Verification items for this drawing (mm, ordinates from the low corner). A direction names the side the tool comes from. Give positions to 0.01 mm unless a question says otherwise; leave off trailing zeros. Write each loop counter-clockwise with the first axis right and the second up, starting at its lowest first coordinate (ties: lowest second). Pieces come first, ordered by that corner, then holes. Notation, with made-up numbers: (5, 59) -> (59, 59) arc R22 ccw to (59, 93) -> close; hole circle Ø4 at (68, 61). An arc over 180 degrees is marked (long way). Write item = value, one per line.
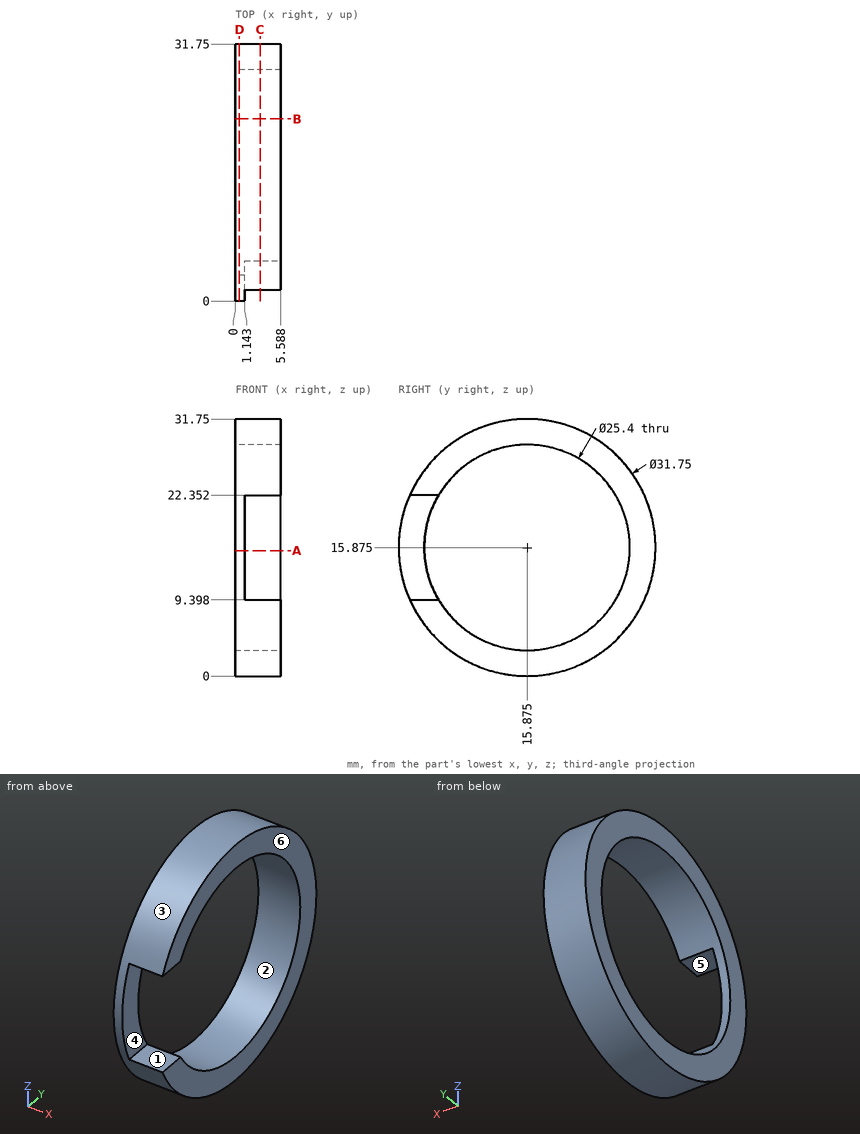
Item 1: Sectioned sample at B-B on y = 22.5. Record the cut outline in (x, z), then the cut area to 3 significant figures.
Response values:
outline = (0, 1.45) -> (5.59, 1.45) -> (5.59, 5.04) -> (0, 5.04) -> close; (0, 26.71) -> (5.59, 26.71) -> (5.59, 30.3) -> (0, 30.3) -> close
area = 40.1 mm^2
Item 2: Sectioned sample at C-C on x = 3.05. Record the cut outline in (y, z) (3 decimals), then the cut area to 3 significant figures.
Response values:
outline = (1.381, 9.398) arc R15.875 ccw (long way) to (1.381, 22.352) -> (4.951, 22.352) arc R12.7 cw (long way) to (4.951, 9.398) -> close
area = 242 mm^2
Item 3: Mould release check, pull along Z, two halves, no side actions. Record for the marked faces 3, 4, 5 and 6: +Z half, -Z half, draft (parallel to the pull), parting line (faces both ways), or undercut.
Response values:
face_3 = parting line
face_4 = undercut
face_5 = undercut
face_6 = draft
Item 4: Sectioned sample at D-D on x = 0.5. Record the cut outline in (y, z) (3 decimals), then the cut area to 3 significant figures.
Response values:
outline = circle Ø31.75 at (15.875, 15.875); hole circle Ø25.4 at (15.875, 15.875)
area = 285 mm^2
Item 5: Material ranges on line 1 (Z direction, x = 1.9, y = 16); line 2 (Z direction, x = 1.8, y = 2); line 3 (Y direction, x = 0.7, z = 13), recorded low to high.
Response values:
line_1 = 0 to 3.18, 28.57 to 31.75
line_2 = 8.16 to 9.4, 22.35 to 23.59
line_3 = 0.26 to 3.5, 28.25 to 31.49
Item 6: Set-up check for the marked faces 1 and 2: record each of +Z, -Z, +X, -X, +Y, -Y from which the full face is reachable in a straight line by a thin tool's end or side.
Response values:
face_1 = +X, -Y
face_2 = +X, -X
Item 7: Sectioned sample at A-A on z = 15.5. Record the cut outline in (x, y), then the cut area to 3 significant figures.
Response values:
outline = (0, 0) -> (1.14, 0) -> (1.14, 3.18) -> (0, 3.18) -> close; (0, 28.57) -> (5.59, 28.57) -> (5.59, 31.75) -> (0, 31.75) -> close
area = 21.4 mm^2
Item 8: Go/stop test with flat-tipped pins: P1, Ø4, axis at y = 2, z = 15.5, coming from the +X side; P2, Ø1.1, axis at x = 4, y = 3, coming from the -Z side; P3, Ø1.5, axis at x = 4.5, z = 21, coming from the +Y side. Record where each tip stops, or that it passes through.
Response values:
P1 = 1.14
P2 = 5.87
P3 = 31.14
